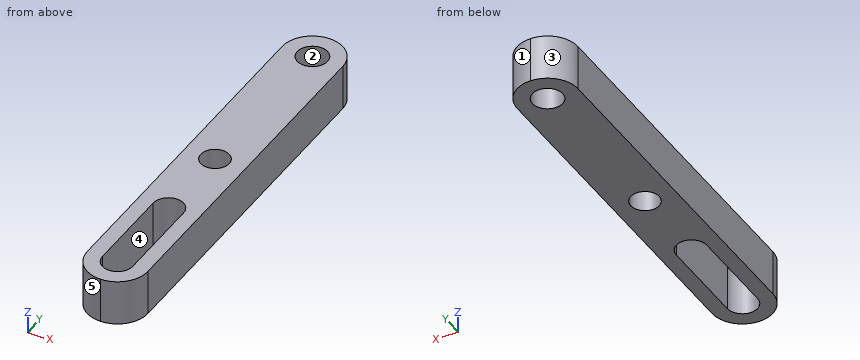
from build123d import *

# Parameters (mm, degrees)
SKETCH1_W           = 6.35
SKETCH1_H           = 42.8625
BOSS_EXTRUDE1_DEPTH = 4.7625
SKETCH2_R           = 1.49225
CUT_EXTRUDE1_DEPTH  = 23.182436922
SKETCH3_R           = 1.5875
CUT_EXTRUDE2_DEPTH  = 23.182436922
FILLET1_R           = 3.175


with BuildPart() as part:
    # Sketch1 → Boss-Extrude1 (new body)
    with BuildSketch(Plane.XY):
        Rectangle(SKETCH1_W, SKETCH1_H)
    extrude(amount=BOSS_EXTRUDE1_DEPTH)

    # Sketch2 → Cut-Extrude1 (cut, through all)
    with BuildSketch(Plane.XY.offset(4.7625)):
        Circle(SKETCH2_R)
    extrude(amount=-CUT_EXTRUDE1_DEPTH, mode=Mode.SUBTRACT)

    # Sketch3 → Cut-Extrude2 (cut, through all)
    with BuildSketch(Plane.XY.offset(4.7625)):
        with Locations((0, 18.25625)):
            Circle(SKETCH3_R)
        with BuildLine():
            Line((1.5875, -18.25625), (1.5875, -8.73125))
            ThreePointArc((1.5875, -8.73125), (0, -7.14375), (-1.5875, -8.73125))
            Line((-1.5875, -8.73125), (-1.5875, -18.25625))
            ThreePointArc((-1.5875, -18.25625), (0, -19.84375), (1.5875, -18.25625))
        make_face()
    extrude(amount=-CUT_EXTRUDE2_DEPTH, mode=Mode.SUBTRACT)

    # Fillet1
    fillet1_edges = [part.edges().sort_by_distance(p)[0] for p in [
        (-3.175, 21.43125, 2.38125),
        (3.175, 21.43125, 2.38125),
        (-3.175, -21.43125, 2.38125),
        (3.175, -21.43125, 2.38125),
    ]]
    fillet(fillet1_edges, radius=FILLET1_R - 0.0001)  # a hair under: the kernel refuses the full size


solid = part.part
Check sheet for the modelled part. Datum: model origin and axes. Units: mm. Face numbers are marked on the shaded views. A direction names the side the tool comes from. Round coordinates to 2 decimals unless told otherwise and drop trailing zeros. Order: outer loops, then holes, each group sorted by start corner. A loop starts at its lowest first (then second) coordinate and runs counter-clockwise, first axis right, second up. Notation, with made-up numbers: M 34.25,-3 L 78.25,-3 A23 ccw 78.25,28 Z; hole C 34,-25 d4. An arc over 180 degrees is marked long. One line per item, written item: value. Start each with the question number.
1. Release check for a two-part mould opening along X. For the marked faces 1, 2 and 3 record: released by +X, released by -X, zero draft, split by the parting line, or undercut.
2. Access from +Z, -Z, +X, -X, +Y, -Y to the whole of each face (thin tool, end or side, straight path). Record for the marked faces 4 and 5.
3. Section check B-B on x = 0.5. Enter the section's corners in (y, z).
4. Section check A-A on y = -11. Enter the section's corners in (x, z) (1 decimal), and give its area (3 significant figures).
5. Scan lines: line 1 along Y through (x, z) = (0, 1.9); line 2 along X through (y, z) = (-17, 1.25) (1 decimal); line 3 along Y through (x, z) = (-1, 0.4). Record each from-to range of solid material in increasing order.
6. Section check D-D on y = 0. Enter the section's corners in (x, z) (1 decimal), and give its area (3 significant figures).
7. Section check C-C on z = 1.55. Give the number of separate pieces and of enclosed holes in the cut face, and give its area (3 significant figures).
Results found:
1. face 1: released by +X
1. face 2: undercut
1. face 3: released by -X
2. face 4: +Z, -Z
2. face 5: +Z, -Z, -X, -Y
3. outline: M -21.39,0 L -19.76,0 L -19.76,4.76 L -21.39,4.76 Z; M -7.22,0 L -1.41,0 L -1.41,4.76 L -7.22,4.76 Z; M 1.41,0 L 16.75,0 L 16.75,4.76 L 1.41,4.76 Z; M 19.76,0 L 21.39,0 L 21.39,4.76 L 19.76,4.76 Z
4. outline: M -3.2,0 L -1.6,0 L -1.6,4.8 L -3.2,4.8 Z; M 1.6,0 L 3.2,0 L 3.2,4.8 L 1.6,4.8 Z
4. area: 15.1 mm^2
5. line 1: -21.43 to -19.84, -7.14 to -1.49, 1.49 to 16.67, 19.84 to 21.43
5. line 2: -3.2 to -1.6, 1.6 to 3.2
5. line 3: -21.27 to -19.49, -7.5 to -1.11, 1.11 to 17.02, 19.49 to 21.27
6. outline: M -3.2,0 L -1.5,0 L -1.5,4.8 L -3.2,4.8 Z; M 1.5,0 L 3.2,0 L 3.2,4.8 L 1.5,4.8 Z
6. area: 16.0 mm^2
7. separate pieces: 1
7. enclosed holes: 3
7. area: 210 mm^2
